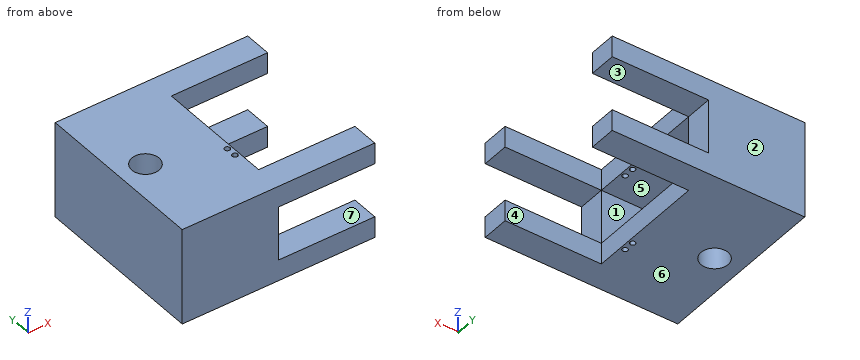
from build123d import *

# Parameters (mm, degrees)
SKETCH1_W             = 12.7
SKETCH1_H             = 9.906
BOSS_EXTRUDE1_DEPTH   = 90
BOSS_EXTRUDE1_2_DEPTH = 90
BOSS_EXTRUDE1_3_DEPTH = 90
BOSS_EXTRUDE1_4_DEPTH = 90
SKETCH1_4_W           = 55.88
SKETCH1_4_H           = 9.906
SKETCH1_4_W_2         = 12.7
SKETCH1_4_H_2         = 25.4
BOSS_EXTRUDE2_DEPTH   = 45
SKETCH1_5_W           = 55.88
SKETCH1_5_H           = 25.4
BOSS_EXTRUDE3_DEPTH   = 5
CUT_EXTRUDE1_DEPTH    = 130.423967425


with BuildPart() as part:
    # Sketch1 → Boss-Extrude1 (new body)
    with BuildSketch(Plane.YZ):
        with Locations((74.93, 4.953)):
            Rectangle(SKETCH1_W, SKETCH1_H)
    extrude(amount=BOSS_EXTRUDE1_DEPTH)



with BuildPart() as body_2:
    # Sketch1 → Boss-Extrude1 2 (new body)
    with BuildSketch(Plane.YZ):
        with Locations((6.35, 40.259)):
            Rectangle(SKETCH1_W, SKETCH1_H)
    extrude(amount=BOSS_EXTRUDE1_2_DEPTH)


with BuildPart() as body_3:
    # Sketch1 → Boss-Extrude1 3 (new body)
    with BuildSketch(Plane.YZ):
        with Locations((6.35, 4.953)):
            Rectangle(SKETCH1_W, SKETCH1_H)
    extrude(amount=BOSS_EXTRUDE1_3_DEPTH)


with BuildPart() as body_4:
    # Sketch1 → Boss-Extrude1 4 (new body)
    with BuildSketch(Plane.YZ):
        with Locations((74.93, 40.259)):
            Rectangle(SKETCH1_W, SKETCH1_H)
    extrude(amount=BOSS_EXTRUDE1_4_DEPTH)


with BuildPart() as part_1:
    add(part.part)

    add(body_2.part)  # Boss-Extrude2 merges body 2

    add(body_3.part)  # Boss-Extrude2 merges body 3

    add(body_4.part)  # Boss-Extrude2 merges body 4
    # Sketch1_4 → Boss-Extrude2 (add)
    with BuildSketch(Plane.YZ):
        with Locations((40.64, 40.259)):
            Rectangle(SKETCH1_4_W, SKETCH1_4_H)
        with Locations((6.35, 22.606)):
            Rectangle(SKETCH1_4_W_2, SKETCH1_4_H_2)
        with Locations((74.93, 22.606)):
            Rectangle(SKETCH1_4_W_2, SKETCH1_4_H_2)
        with Locations((40.64, 4.953)):
            Rectangle(SKETCH1_4_W, SKETCH1_4_H)
    extrude(amount=BOSS_EXTRUDE2_DEPTH)

    # Sketch1_5 → Boss-Extrude3 (add)
    with BuildSketch(Plane.YZ):
        with Locations((40.64, 22.606)):
            Rectangle(SKETCH1_5_W, SKETCH1_5_H)
    extrude(amount=BOSS_EXTRUDE3_DEPTH)

    # Sketch3 → Cut-Extrude1 (cut, through all)
    with BuildSketch(Plane.XY.offset(45.212)):
        with BuildLine():
            ThreePointArc((43, 28.73), (43.898025612, 29.101974388), (44.27, 30))
            Line((44.27, 30), (43, 30))
            Line((43, 30), (43, 28.73))
        make_face()
        with BuildLine():
            Line((43, 28.73), (43, 30))
            Line((43, 30), (41.73, 30))
            ThreePointArc((41.73, 30), (42.101974388, 29.101974388), (43, 28.73))
        make_face()
        with BuildLine():
            Line((43, 30), (44.27, 30))
            ThreePointArc((44.27, 30), (43, 31.27), (41.73, 30))
            Line((41.73, 30), (43, 30))
        make_face()
        with BuildLine():
            ThreePointArc((6.15, 40.64), (12.5, 34.29), (18.85, 40.64))
            Line((18.85, 40.64), (6.15, 40.64))
        make_face()
        with BuildLine():
            Line((6.15, 40.64), (18.85, 40.64))
            ThreePointArc((18.85, 40.64), (12.5, 46.99), (6.15, 40.64))
        make_face()
        with BuildLine():
            ThreePointArc((44.27, 25.1359), (43.898025612, 26.033925612), (43, 26.4059))
            Line((43, 26.4059), (43, 25.1359))
            Line((43, 25.1359), (43, 23.8659))
            ThreePointArc((43, 23.8659), (43.898025612, 24.237874388), (44.27, 25.1359))
        make_face()
        with BuildLine():
            Line((43, 25.1359), (43, 26.4059))
            ThreePointArc((43, 26.4059), (41.73, 25.1359), (43, 23.8659))
            Line((43, 23.8659), (43, 25.1359))
        make_face()
    extrude(amount=-CUT_EXTRUDE1_DEPTH, mode=Mode.SUBTRACT)


solid = part_1.part
Input: part model. Units: mm. Frame: model coordinates. Face numbers are marked on the shaded views. A direction names the side the tool comes from. Give positions to 0.01 mm unless a question says otherwise; leave off trailing zeros. Write each loop counter-clockwise with the first axis right and the second up, starting at its lowest first coordinate (ties: lowest second). Pieces come first, ordered by that corner, then holes.
Q1. Pull-direction query (Y, two-part tool) for the marked faces 1, 2 and 3; classes: pulls with the +Y half, pulls with the -Y half, needs draft (parallel to the pull), parting line crosses it, or undercut.
Q2. Set-up query: the marked faces 4, 5, 6 and 7. Return all of +Z, -Z, +X, -X, +Y, -Y with unobstructed straight access to the full face (end or side cutting, diameter ignored); none if empty.
Q3. Material intervals for probe 1 along Z at (x, y) = (17, 35); probe 2 along Y at (x, z) = (43, 19); probe 3 along Y at (x, z) = (12.5, 41.25), sorted ascending.
Q4. Section A-A, the plane x = 76. Output: boundary loops of the cut face in (y, z), plus the area to 3 significant figures.
Q5. First-contact query: P1, Ø4, axis at y = 77, z = 21, coming from the +X side; P2, Ø2, axis at x = 56.5, z = 11, coming from the +Y side; P3, Ø11, axis at x = 71.5, z = 42, coming from the -Y side. Flat tips, straight axial feed; report the tip coordinate or a pass-through.
Q6. Section D-D, the plane z = 40.5. Output: boundary loops of the cut face in (x, y).
Q7. Section C-C, the plane x = 12.5. Output: boundary loops of the cut face in (y, z).
Q8. Section B-B, the plane z = 21. Output: boundary loops of the cut face in (x, y), plus the area to 3 significant figures.
Filled in:
1. face 1: undercut
1. face 2: pulls with the +Y half
1. face 3: needs draft
2. face 4: +Z, -Z, +X
2. face 5: +X
2. face 6: -Z, +X, -X, +Y, -Y
2. face 7: +X, +Y, -Y
3. probe 1: z = 0 to 9.91, 35.31 to 45.21
3. probe 2: y = 0 to 12.7, 68.58 to 81.28
3. probe 3: y = 0 to 34.29, 46.99 to 81.28
4. outline: (0, 0) - (12.7, 0) - (12.7, 9.91) - (0, 9.91) - close; (0, 35.31) - (12.7, 35.31) - (12.7, 45.21) - (0, 45.21) - close; (68.58, 0) - (81.28, 0) - (81.28, 9.91) - (68.58, 9.91) - close; (68.58, 35.31) - (81.28, 35.31) - (81.28, 45.21) - (68.58, 45.21) - close
4. area: 503 mm2
5. P1: stops at x = 45
5. P2: passes through
5. P3: stops at y = 0
6. outline: (0, 0) - (90, 0) - (90, 12.7) - (45, 12.7) - (45, 68.58) - (90, 68.58) - (90, 81.28) - (0, 81.28) - close; hole circle Ø12.7 at (12.5, 40.64); hole circle Ø2.54 at (43, 25.14); hole circle Ø2.54 at (43, 30)
7. outline: (0, 0) - (34.29, 0) - (34.29, 9.91) - (12.7, 9.91) - (12.7, 35.31) - (34.29, 35.31) - (34.29, 45.21) - (0, 45.21) - close; (46.99, 0) - (81.28, 0) - (81.28, 45.21) - (46.99, 45.21) - (46.99, 35.31) - (68.58, 35.31) - (68.58, 9.91) - (46.99, 9.91) - close
8. outline: (0, 0) - (45, 0) - (45, 12.7) - (5, 12.7) - (5, 68.58) - (45, 68.58) - (45, 81.28) - (0, 81.28) - close
8. area: 1,420 mm2
